Read the model definition and answer for the solid it produces. Units are mm, in the model's axes. Face numbers are marked on the shaded views. A direction names the side the tool comes from. Coordinates: 2 decimals unless noted, no trailing zeros. Write each loop counter-clockwise with the first axis right and the second up, starting at its lowest first coordinate (ties: lowest second). Pieces come first, ordered by that corner, then holes. Notation, with made-up numbers: (14.5, -3) -> (32.5, -3) arc R3 ccw to (32.5, 1) -> close; hole circle Ø11 at (-20.5, 68). An arc over 180 degrees is marked (long way). One line per item, written item: value. Start each with the question number.
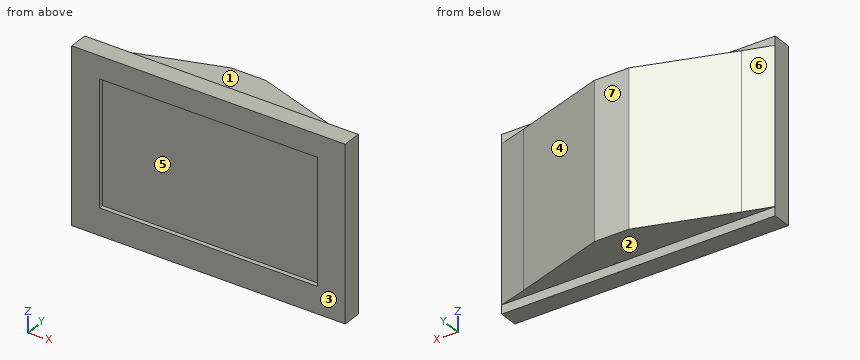
from build123d import *

# Parameters (mm, degrees)
F0_W          = 123
F0_H          = 78
F1_DEPTH      = 8.5
F2_W          = 98
F2_H          = 56
F3_DEPTH      = 2
F5_DEPTH      = 35
F5_DEPTH_BACK = 35


with BuildPart() as f1:
    # F0 (on Front) → F1 (new body)
    with BuildSketch(Plane.XZ):
        Rectangle(F0_W, F0_H)
    extrude(amount=-F1_DEPTH)

    # F2 (on face) → F3 (cut)
    with BuildSketch(Plane.XZ):
        with Locations((0, 1)):
            Rectangle(F2_W, F2_H)
    extrude(amount=-F3_DEPTH, mode=Mode.SUBTRACT)

    # F4 (on Top) → F5 (join, two sides)
    with BuildSketch(Plane.XY) as f5_sk:
        Polygon((-49, 12.4), (-61.5, 8.5), (61.5, 8.5), (49, 12.4), (7.791058, 26), (0, 26), (-7.791058, 26), align=None)
    extrude(amount=F5_DEPTH)
    extrude(f5_sk.sketch, amount=-F5_DEPTH_BACK)


solid = f1.part
1. A cutting plane is placed at D-D on x = 52.5. Give the vertices of the cut face in (y, z), then the cut area to 3 significant figures.
2. A cutting plane is placed at A-A on z = 32.5. Give the vertices of the cut face in (x, y).
3. For a pull along X with two mould halves and no side action, classify the marked faces 4, 5, 6 and 7 as +X half, -X half, draft (parallel to the pull), parting line (faces both ways), or undercut.
4. A tool of negligible diameter and unlimited length cuts with its end or side. For the marked faces 1, 2 and 3, from which of +Z, -Z, +X, -X, +Y, -Y can it reach the whole face along a straight path? Write none if from no direction.
5. A cutting plane is placed at C-C on y = 17.5. Give the vertices of the cut face in (x, z).
6. A cutting plane is placed at B-B on x = -2.5. Give the vertices of the cut face in (y, z).
7. Find the intervals of material crossed by probe 1 along Z at (x, y) = (-32, 1.5); probe 2 along X at (y, z) = (1.75, 19); probe 3 along Z at (x, y) = (37, 11.5), in increasing order. Write a range as from..to.
8. Given pin 1 (14 mm diameter, centred on x = 27.5, y = 19, fed in from -Z); pin 2 (4 mm diameter, centred on x = 28.5, z = -1.5, fed in from -Y); pin 3 (10 mm diameter, centred on x = 29, z = 14, fed in from +Y), each flat-ended and moving along its own axis, determine where each tip first touches the part or whether it passes through.
Derived:
1. outline: (0, -39) -> (8.5, -39) -> (8.5, -35) -> (11.31, -35) -> (11.31, 35) -> (8.5, 35) -> (8.5, 39) -> (0, 39) -> close
1. area: 860 mm2
2. outline: (-61.5, 0) -> (61.5, 0) -> (61.5, 8.5) -> (49, 12.4) -> (7.79, 26) -> (-7.79, 26) -> (-49, 12.4) -> (-61.5, 8.5) -> close
3. face 4: +X half
3. face 5: undercut
3. face 6: -X half
3. face 7: draft
4. face 1: +Z, +X, -X, +Y
4. face 2: -Z, +X, -X, +Y
4. face 3: +Z, -Z, +X, -X, -Y
5. outline: (-33.55, -35) -> (33.55, -35) -> (33.55, 35) -> (-33.55, 35) -> close
6. outline: (0, -39) -> (8.5, -39) -> (8.5, -35) -> (26, -35) -> (26, 35) -> (8.5, 35) -> (8.5, 39) -> (0, 39) -> (0, 29) -> (2, 29) -> (2, -27) -> (0, -27) -> close
7. probe 1: z = -39..-27, 29..39
7. probe 2: x = -61.5..-49, 49..61.5
7. probe 3: z = -35..35
8. pin 1: stops at z = -35
8. pin 2: stops at y = 2
8. pin 3: stops at y = 20.65
